CAD build for the part. Positions are in the model's coordinates, mm. Coordinates: 2 decimals unless noted, no trailing zeros. Loops run counter-clockwise (first coordinate to the right, second up) from the corner with the lowest first, then second, coordinate; pieces in that order, holes last. Notation, with made-up numbers: (5.25, -14) - (28.25, -14) arc R34 cw to (28.25, 22) - close; hole circle Ø11 at (14, 57). An arc over 180 degrees is marked (long way). Put each result on its own line as item: value.
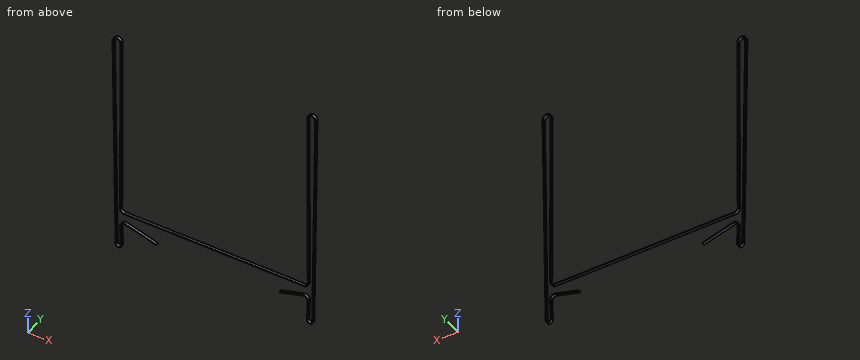
```python
from build123d import *

# Parameters (mm, degrees)
EXTRUDE_THIN1_START = 98.137598
EXTRUDE_THIN1_DEPTH = 6.35


with BuildPart() as part:
    # Sketch1 → Extrude-Thin1 (new body)
    with BuildSketch(Plane(origin=(0, 0, 0), x_dir=(1, 0, 0), z_dir=(0, 1, 0)).offset(EXTRUDE_THIN1_START)):
        with BuildLine():
            Line((400.023485906, -85.443361152), (454.971450984, -101.27596863))
            ThreePointArc((454.971450984, -101.27596863), (463.861362415, -99.548472953), (467.668957804, -91.331601045))
            Line((467.668957804, -91.331601045), (465.755105618, -41.69369751))
            ThreePointArc((465.755105618, -41.69369751), (471.16659983, -35.920320597), (476.872500072, -41.402916061))
            Line((476.872500072, -41.402916061), (484.032084809, -561.613939409))
            ThreePointArc((484.032084809, -561.613939409), (475.331383816, -570.484218666), (466.532944878, -561.710876992))
            Line((466.532944878, -561.710876992), (467.676291292, -135.561743547))
            ThreePointArc((467.676291292, -135.561743547), (464.771471532, -128.508780211), (457.726327103, -125.585048067))
            Line((457.726327103, -125.585048067), (217.954761626, -125.585048067))
            Line((217.954761626, -125.585048067), (34.733672902, -125.585048067))
            ThreePointArc((34.733672902, -125.585048067), (27.688528473, -128.508780211), (24.783708713, -135.561743547))
            Line((24.783708713, -135.561743547), (25.927055127, -561.710876992))
            ThreePointArc((25.927055127, -561.710876992), (17.128616189, -570.484218666), (8.427915196, -561.613939409))
            Line((8.427915196, -561.613939409), (15.587499933, -41.402916061))
            ThreePointArc((15.587499933, -41.402916061), (21.293400175, -35.920320597), (26.704894387, -41.69369751))
            Line((26.704894387, -41.69369751), (24.791042201, -91.331601045))
            ThreePointArc((24.791042201, -91.331601045), (28.59863759, -99.548472953), (37.488549021, -101.27596863))
            Line((37.488549021, -101.27596863), (109.817026065, -80.435371805))
            Line((109.817026065, -80.435371805), (109.4847775, -79.282284258))
            Line((109.4847775, -79.282284258), (37.156300457, -100.122881082))
            ThreePointArc((37.156300457, -100.122881082), (29.338539147, -98.603726593), (25.990151243, -91.377834212))
            Line((25.990151243, -91.377834212), (27.904003429, -41.739930677))
            ThreePointArc((27.904003429, -41.739930677), (21.324776092, -34.720730854), (14.387613566, -41.386402209))
            Line((14.387613566, -41.386402209), (7.22802883, -561.597425557))
            ThreePointArc((7.22802883, -561.597425557), (17.121968816, -571.684200254), (27.127050808, -561.707657437))
            Line((27.127050808, -561.707657437), (25.983704394, -135.558523992))
            ThreePointArc((25.983704394, -135.558523992), (28.538194133, -129.356169299), (34.733672902, -126.785048067))
            Line((34.733672902, -126.785048067), (217.954761626, -126.785048067))
            Line((217.954761626, -126.785048067), (457.726327103, -126.785048067))
            ThreePointArc((457.726327103, -126.785048067), (463.921805872, -129.356169299), (466.476295611, -135.558523992))
            Line((466.476295611, -135.558523992), (465.332949197, -561.707657437))
            ThreePointArc((465.332949197, -561.707657437), (475.338031189, -571.684200254), (485.231971175, -561.597425557))
            Line((485.231971175, -561.597425557), (478.072386439, -41.386402209))
            ThreePointArc((478.072386439, -41.386402209), (471.135223913, -34.720730854), (464.555996576, -41.739930677))
            Line((464.555996576, -41.739930677), (466.469848762, -91.377834212))
            ThreePointArc((466.469848762, -91.377834212), (463.121460857, -98.603726593), (455.303699548, -100.122881082))
            Line((455.303699548, -100.122881082), (400.355734471, -84.290273604))
            Line((400.355734471, -84.290273604), (400.023485906, -85.443361152))
        make_face()
    extrude(amount=EXTRUDE_THIN1_DEPTH)


solid = part.part
```
Q1. Slice it at B-B, the plane x = 78.5. Give the cut face in (y, z).
Determined:
outline: (98.14, 88.21) - (104.49, 88.21) - (104.49, 89.46) - (98.14, 89.46) - close; (98.14, 125.59) - (104.49, 125.59) - (104.49, 126.79) - (98.14, 126.79) - close
Q2. Pin check, flat tips, straight feed: pin 1 Ø1.5 at (x, y) = (172, 102) entering from +Z; pin 2 Ø1 at (y, z) = (99, 453) entering from -X; pin 3 Ø1.9 at (x, y) = (217, 101) entering from -Z. Stop position of each tip, or through.
Determined:
pin 1: z = 126.79
pin 2: x = 8.72
pin 3: z = 125.59
Q3. Slice it at A-A, the plane z = 274. Give the cut face in (x, y), then the cut area to 3 significant figures.
Determined:
outline: (11.19, 98.14) - (12.39, 98.14) - (12.39, 104.49) - (11.19, 104.49) - close; (25.16, 98.14) - (26.36, 98.14) - (26.36, 104.49) - (25.16, 104.49) - close; (466.1, 98.14) - (467.3, 98.14) - (467.3, 104.49) - (466.1, 104.49) - close; (480.07, 98.14) - (481.27, 98.14) - (481.27, 104.49) - (480.07, 104.49) - close
area: 30.5 mm2
Q4. Slice it at D-D, the plane x = 326. Give the cut face in (y, z).
Determined:
outline: (98.14, 125.59) - (104.49, 125.59) - (104.49, 126.79) - (98.14, 126.79) - close
Q5. Slice it at C-C, the plane z = 114.5. Give the cut face in (x, y).
Determined:
outline: (13.38, 98.14) - (14.58, 98.14) - (14.58, 104.49) - (13.38, 104.49) - close; (477.88, 98.14) - (479.08, 98.14) - (479.08, 104.49) - (477.88, 104.49) - close
Q6. Wall check: L1, parallel to X at y = 100, z = 236; L2, parallel to X at y = 98.5, z = 252.5; L3, parallel to Z at x = 320, y = 104. Give the ranges that are in metal, low to high. Write a range as from..to.
Determined:
L1: 11.71..12.91, 25.05..26.25, 466.21..467.41, 479.55..480.75
L2: 11.48..12.68, 25.1..26.3, 466.16..467.36, 479.78..480.98
L3: 125.59..126.79
